Input: dimensioned drawing with shaded views. Units: mm. Origin: part minimum x, y, z. Round coordinates to 2 decimals unless told otherwise and drop trailing zeros. Order: outer loops, then holes, each group sorted by start corner. A loop starts at its lowest first (then second) coordinate and runs counter-clockwise, first axis right, second up. Notation, with made-up numbers: (73.25, -27) -> (104.25, -27) arc R23 ccw to (104.25, 1) -> close; hole circle Ø4 at (86, 53). An arc over 180 degrees is marked (long way). Use a Markdown table: item, result. Add a question column.
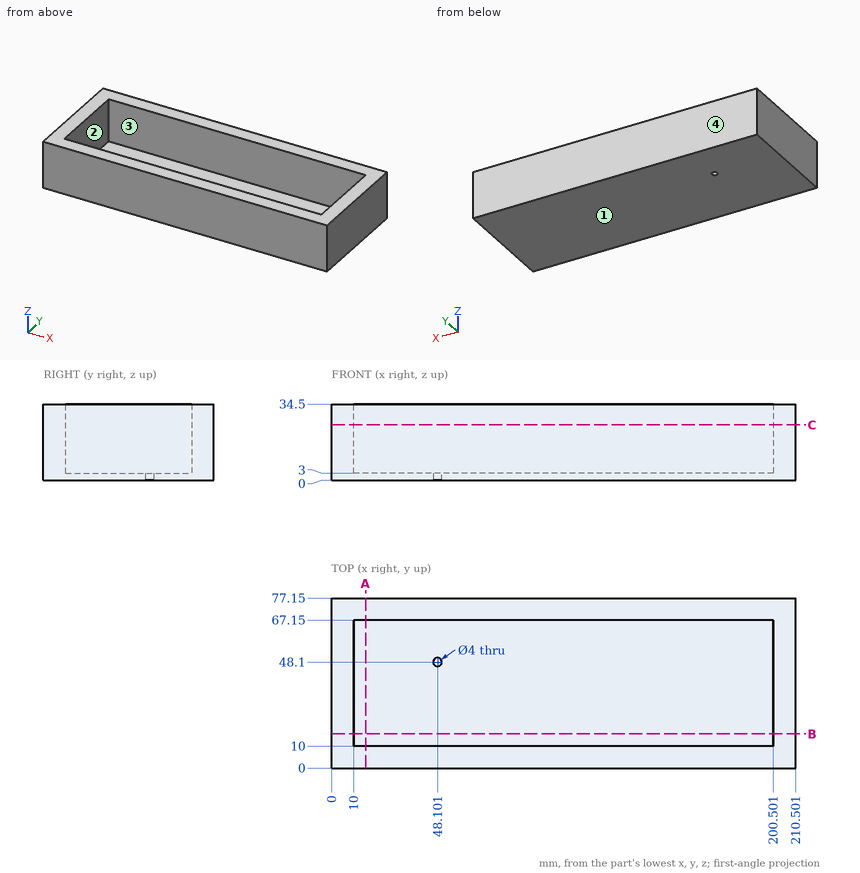
1) Section B-B on y = 15.5. Output: boundary loops of the cut face in (x, z), then the cut area to 3 significant figures.
2) Draft query along Y for the marked faces 1, 2, 3 and 4. Return one class per face: pulls with the +Y half, pulls with the -Y half, needs draft (parallel to the pull), parting line crosses it, or undercut.
3) Line query: probe 1 along X at (y, z) = (51.5, 9); probe 2 along Y at (x, z) = (67.5, 26.5); probe 3 along Z at (x, y) = (175, 37). Output: solid intervals per line, ascending. Write a range as from..to.
4) First-contact query: pin 1 Ø2.5 at (x, y) = (48.1, 48.1) entering from +Z; pin 2 Ø1 at (x, y) = (37, 41) entering from +Z. Flat tips, straight axial feed; report the tip coordinate or a pass-through.
5) Section C-C on z = 25. Output: boundary loops of the cut face in (x, y).
6) Section A-A on x = 15.5. Output: boundary loops of the cut face in (y, z).
Conclusion:
| question | item | result |
|---|---|---|
| 1 | outline | (0, 0) -> (210.5, 0) -> (210.5, 34.5) -> (200.5, 34.5) -> (200.5, 3) -> (10, 3) -> (10, 34.5) -> (0, 34.5) -> close |
| 1 | area | 1,260 mm^2 |
| 2 | face 1 | needs draft |
| 2 | face 2 | undercut |
| 2 | face 3 | undercut |
| 2 | face 4 | pulls with the +Y half |
| 3 | probe 1 | x = 0..10, 200.5..210.5 |
| 3 | probe 2 | y = 0..10, 67.15..77.15 |
| 3 | probe 3 | z = 0..3 |
| 4 | pin 1 | passes through |
| 4 | pin 2 | stops at z = 3 |
| 5 | outline | (0, 0) -> (210.5, 0) -> (210.5, 77.15) -> (0, 77.15) -> close; hole (10, 10) -> (200.5, 10) -> (200.5, 67.15) -> (10, 67.15) -> close |
| 6 | outline | (0, 0) -> (77.15, 0) -> (77.15, 34.5) -> (67.15, 34.5) -> (67.15, 3) -> (10, 3) -> (10, 34.5) -> (0, 34.5) -> close |
